```python
from build123d import *

# Parameters (mm, degrees)
F0_W     = 77
F0_H     = 24
F0_R     = 2.5
F1_DEPTH = 1.5
F2_W     = 3
F2_H     = 9
F3_DEPTH = 3
F4_SIZE  = 2.99999


# Not quite as in the source:
# - a fillet or chamfer is up to 0.001 mm smaller than in the source, because OpenCascade refuses the exact size


with BuildPart() as f1:
    # F0 (on Top) → F1 (new body)
    with BuildSketch(Plane.XY):
        Rectangle(F0_W, F0_H)
        with Locations((-29.5, 0)):
            Circle(F0_R, mode=Mode.SUBTRACT)
        Polygon((-35.5, -5), (-35.5, 5), (-15, 5), (-15, 4.5), (-35, 4.5), (-35, -4.5), (-15, -4.5), (-15, -5), align=None, mode=Mode.SUBTRACT)
        with BuildLine():
            Line((18.5, 4), (18.5, 8))
            Line((18.5, 8), (19.5, 8))
            Line((19.5, 8), (19.5, -8))
            Line((19.5, -8), (18.5, -8))
            Line((18.5, -8), (18.5, -4))
            ThreePointArc((18.5, -4), (14.5, 0), (18.5, 4))
        make_face(mode=Mode.SUBTRACT)
    extrude(amount=F1_DEPTH)

    # F2 (on face) → F3 (join)
    with BuildSketch(Plane.XY.offset(1.5)):
        with Locations((-33.5, 0)):
            Rectangle(F2_W, F2_H)
    extrude(amount=F3_DEPTH)

    # F4 (size 3 in the source; OpenCascade refuses exactly that, so slightly less here)
    f4_edges = [f1.edges().sort_by_distance(p)[0] for p in [
        (-32, 0, 4.5),
    ]]
    chamfer(f4_edges, length=F4_SIZE)


solid = f1.part
```
Design review of the part built by this model. Coordinates are the model's own, in mm. A direction names the side the tool comes from. Round coordinates to 2 decimals unless told otherwise and drop trailing zeros. Write each loop counter-clockwise with the first axis right and the second up, starting at its lowest first coordinate (ties: lowest second). Pieces come first, ordered by that corner, then holes. Notation, with made-up numbers: (17, 17) -> (55, 17) arc R21 ccw to (55, 50) -> close; hole circle Ø6 at (22.5, 3). An arc over 180 degrees is marked (long way). Answer in a Markdown table with one row per item.
Q1. Take a section at D-D, the plane x = 4. State the section outline as (y, z) points.
The answers:
| item | result |
|---|---|
| outline | (-12, 0) -> (12, 0) -> (12, 1.5) -> (-12, 1.5) -> close |
Q2. Take a section at A-A, the plane x = -29.5. State the section outline as (y, z) points, then the cut area to 3 significant figures.
The answers:
| item | result |
|---|---|
| outline | (-12, 0) -> (-5, 0) -> (-5, 1.5) -> (-12, 1.5) -> close; (-4.5, 0) -> (-2.5, 0) -> (-2.5, 1.5) -> (-4.5, 1.5) -> close; (2.5, 0) -> (4.5, 0) -> (4.5, 1.5) -> (2.5, 1.5) -> close; (5, 0) -> (12, 0) -> (12, 1.5) -> (5, 1.5) -> close |
| area | 27.0 mm² |
Q3. To check wall thickness, follow L1, parallel to X at y = 0, z = 0.3; L2, parallel to Y at x = -29.5, z = 0.7; L3, parallel to X at y = 1.25, z = 0.7. State the ranges of each line that lie inside material, in increasing order. Write a range as [from, to].
The answers:
| item | result |
|---|---|
| L1 | [-38.5, -35.5], [-35, -32], [-27, 14.5], [19.5, 38.5] |
| L2 | [-12, -5], [-4.5, -2.5], [2.5, 4.5], [5, 12] |
| L3 | [-38.5, -35.5], [-35, -31.67], [-27.33, 14.7], [19.5, 38.5] |
Q4. For faces 1 (the face through (-38.5, 0, 1)), 2 (the face through (-25, -5, 1)), list the 3-axis set-ups (+Z, -Z, +X, -X, +Y, -Y) from which the entire face can be reached by the end or side of a thin tool; tool diameter is ignored.
The answers:
| item | result |
|---|---|
| face 1 | +Z, -Z, -X, +Y, -Y |
| face 2 | +Z, -Z |
Q5. Draft analysis for pull direction X (two halves, no side actions). For faces 3 (the face through (18.5, 6, 1)), 4 (the face through (-1, 12, 1)), 5 (the face through (-33.5, -0.1, 3)), state which applies: +X half, -X half, draft (parallel to the pull), parting line (faces both ways), or undercut.
The answers:
| item | result |
|---|---|
| face 3 | undercut |
| face 4 | draft |
| face 5 | +X half |
Q6. Take a section at C-C, the plane y = -1. Count the separate pieces of the cut face and the enclosed holes in it, then the cut area to 3 significant figures.
The answers:
| item | result |
|---|---|
| separate pieces | 4 |
| enclosed holes | 0 |
| area | 105 mm² |
Q7. Clearance check with a flat-ended pin moving along its axis: pin 1 Ø12 at (x, y) = (21.5, -0.5) entering from +Z. State where the tip first meets the part, or that it passes through.
The answers:
| item | result |
|---|---|
| pin 1 | z = 1.5 |
Q8. Take a section at B-B, the plane y = -6.25. State the section outline as (x, z) points.
The answers:
| item | result |
|---|---|
| outline | (-38.5, 0) -> (18.5, 0) -> (18.5, 1.5) -> (-38.5, 1.5) -> close; (19.5, 0) -> (38.5, 0) -> (38.5, 1.5) -> (19.5, 1.5) -> close |
